```python
from build123d import *

# Parameters (mm, degrees)
ESQUISSE1_W        = 55
ESQUISSE1_H        = 66
ESQUISSE1_R        = 1.5
ESQUISSE1_R_2      = 1
BOSS_EXTRU_1_DEPTH = 3


with BuildPart() as part:
    # Esquisse1 → Boss.-Extru.1 (new body)
    with BuildSketch(Plane(origin=(0, 0, 0), x_dir=(1, 0, 0), z_dir=(0, 1, 0))):
        with Locations((-0.039557044, -0.082747187)):
            Rectangle(ESQUISSE1_W, ESQUISSE1_H)
        with Locations(Location((-25.039557044, 29.917252813, 0), (0, 0, 270))):
            Circle(ESQUISSE1_R, mode=Mode.SUBTRACT)
        with Locations(Location((24.960442956, 29.917252813, 0), (0, 0, 270))):
            Circle(ESQUISSE1_R, mode=Mode.SUBTRACT)
        with Locations(Location((24.960442956, -30.082747187, 0), (0, 0, 270))):
            Circle(ESQUISSE1_R, mode=Mode.SUBTRACT)
        with Locations(Location((-25.039557044, -30.082747187, 0), (0, 0, 270))):
            Circle(ESQUISSE1_R, mode=Mode.SUBTRACT)
        with Locations(Location((15.460442956, 12.917252813, 0), (0, 0, 270))):
            Circle(ESQUISSE1_R_2, mode=Mode.SUBTRACT)
        with Locations(Location((15.460442956, 2.917252813, 0), (0, 0, 270))):
            Circle(ESQUISSE1_R_2, mode=Mode.SUBTRACT)
    extrude(amount=BOSS_EXTRU_1_DEPTH)


solid = part.part
```
Check sheet for the modelled part. Datum: model origin and axes. Units: mm. Give positions to 0.01 mm unless a question says otherwise; leave off trailing zeros. Answer as a JSON object with one key per item and string values. Group by question number.
1) Thickness scan on probe 1 along X at (y, z) = (1.5, -30); probe 2 along Z at (x, y) = (-25, 1.75); probe 3 along Z at (x, y) = (15, 2.6). Record the ranges inside material, lowest first. Write a range as from..to.
2) Depth check by flat-ended pin: P1, Ø1.6, axis at x = 15.46, z = -12.92, coming from the -Y side; P2, Ø3, axis at x = 15.46, z = -2.92, coming from the +Y side. Enter the tip coordinate at first touch or a pass-through.
3) Release check for a two-part mould opening along Z. For faces 1 (the face through (0, 1, 33.083)), 2 (the face through (0, 1, -32.917)), 3 (the face through (16.45, 1.48, -13.05)) record: pulls with the +Z half, pulls with the -Z half, needs draft (parallel to the pull), parting line crosses it, or undercut.
Geometry results:
{
 "1": {"probe 1": "x = -27.54..-26.54, -23.54..23.46, 26.46..27.46", "probe 2": "z = -32.92..-31.42, -28.42..28.58, 31.58..33.08", "probe 3": "z = -32.92..-13.8, -12.03..-3.8, -2.03..33.08"},
 "2": {"P1": "passes through", "P2": "stops at y = 3"},
 "3": {"face 1": "pulls with the +Z half", "face 2": "pulls with the -Z half", "face 3": "undercut"}
}
